Check sheet for the drawn part. Datum: minimum x, y, z corner. Units: mm. A direction names the side the tool comes from. Coordinates: 2 decimals unless noted, no trailing zeros. Order: outer loops, then holes, each group sorted by start corner. A loop starts at its lowest first (then second) coordinate and runs counter-clockwise, first axis right, second up. Notation, with made-up numbers: M 64.25,35 L 103.25,35 A22 cw 103.25,54 Z; hole C 68,-21 d10. An arc over 180 degrees is marked long. Answer in a Markdown table with one row per item. Add a question column.
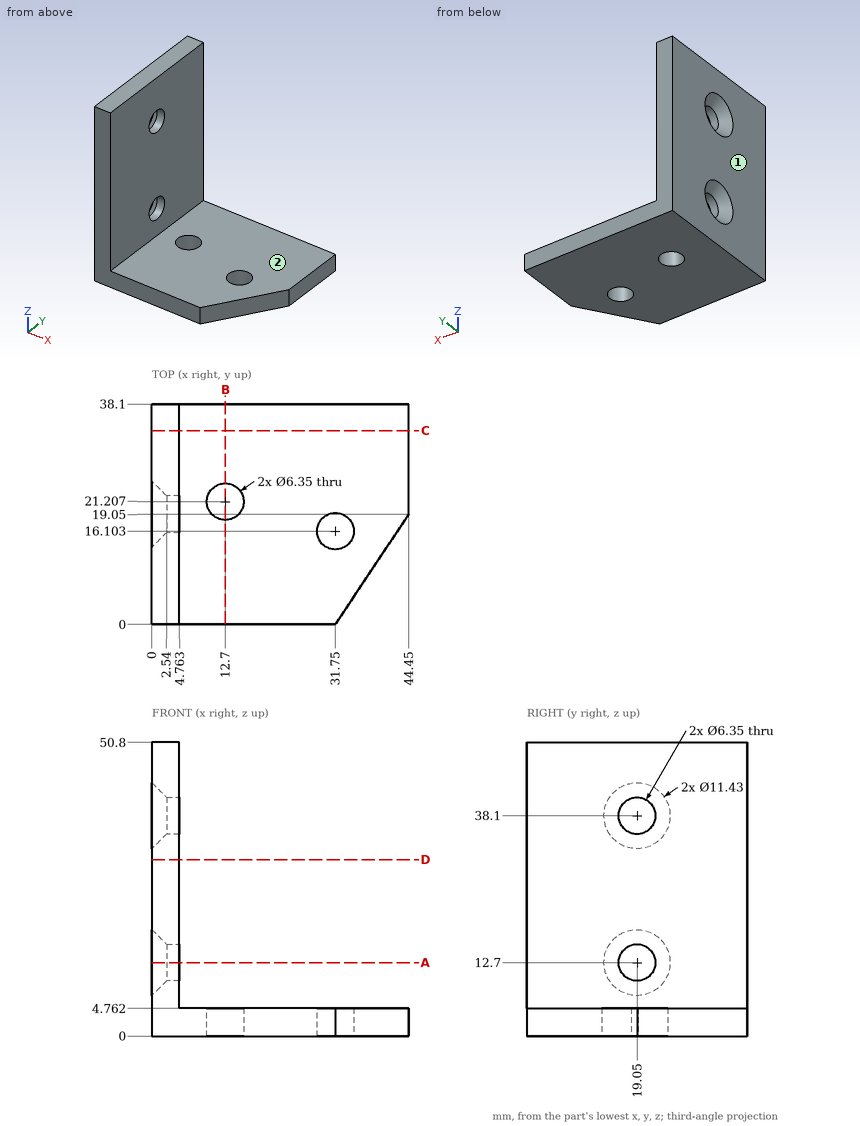
1. Go/stop test with flat-tipped pins: pin 1 Ø4 at (y, z) = (19.5, 16) entering from +X; pin 2 Ø10 at (y, z) = (19.05, 12.7) entering from -X (1 decimal); pin 3 Ø8.5 at (y, z) = (19.05, 38.1) entering from -X (1 decimal). Record where each tip stops, or that it passes through.
2. Section check B-B on x = 12.7. Enter the section's corners in (y, z).
3. Scan lines: line 1 (Z direction, x = 3, y = 19) (1 decimal); line 2 (Y direction, x = 31.75, z = 2.2) (1 decimal); line 3 (Y direction, x = 12.7, z = 2.05). Record each from-to range of solid material in increasing order.
4. Section check D-D on z = 30.5. Enter the section's corners in (x, y).
5. Section check A-A on z = 12.7. Enter the section's corners in (x, y) (1 decimal).
6. Set-up check for the marked faces 1 and 2: record each of +Z, -Z, +X, -X, +Y, -Y from which the full face is reachable in a straight line by a thin tool's end or side.
7. Section check C-C on y = 33.5. Enter the section's corners in (x, z), then the cut area to 3 significant figures.
Result sheet:
| question | item | result |
|---|---|---|
| 1 | pin 1 | x = 4.76 |
| 1 | pin 2 | x = 0.7 |
| 1 | pin 3 | x = 1.5 |
| 2 | outline | M 0,0 L 18.03,0 L 18.03,4.76 L 0,4.76 Z; M 24.38,0 L 38.1,0 L 38.1,4.76 L 24.38,4.76 Z |
| 3 | line 1 | 0 to 9.5, 15.9 to 34.9, 41.3 to 50.8 |
| 3 | line 2 | 0 to 12.9, 19.3 to 38.1 |
| 3 | line 3 | 0 to 18.03, 24.38 to 38.1 |
| 4 | outline | M 0,0 L 4.76,0 L 4.76,38.1 L 0,38.1 Z |
| 5 | outline | M 0,0 L 4.8,0 L 4.8,15.9 L 2.5,15.9 L 0,13.3 Z; M 0,24.8 L 2.5,22.2 L 4.8,22.2 L 4.8,38.1 L 0,38.1 Z |
| 6 | face 1 | +Z, -Z, -X, +Y, -Y |
| 6 | face 2 | +Z, +X, +Y, -Y |
| 7 | outline | M 0,0 L 44.45,0 L 44.45,4.76 L 4.76,4.76 L 4.76,50.8 L 0,50.8 Z |
| 7 | area | 431 mm^2 |
